from build123d import *

# Parameters (mm, degrees)
SKETCH1_R           = 19.05
BOSS_EXTRUDE1_DEPTH = 5.08
SKETCH3_R           = 7.5
BOSS_EXTRUDE2_DEPTH = 7.62
CUT_EXTRUDE1_DEPTH  = 7.62
SKETCH5_R           = 15.494
CUT_EXTRUDE2_DEPTH  = 3.81


with BuildPart() as part:
    # Sketch1 → Boss-Extrude1 (new body)
    with BuildSketch(Plane(origin=(0, 0, 0), x_dir=(1, 0, 0), z_dir=(0, 1, 0))):
        with Locations(Location((0, 0, 0), (0, 0, 270))):
            Circle(SKETCH1_R)
    extrude(amount=BOSS_EXTRUDE1_DEPTH)

    # Sketch3 → Boss-Extrude2 (add)
    with BuildSketch(Plane(origin=(0, 5.08, 0), x_dir=(1, 0, 0), z_dir=(0, 1, 0))):
        with Locations(Location((0, 0, 0), (0, 0, 90))):
            Circle(SKETCH3_R)
    extrude(amount=BOSS_EXTRUDE2_DEPTH)

    # Sketch4 → Cut-Extrude1 (cut)
    with BuildSketch(Plane(origin=(0, 12.7, 0), x_dir=(1, 0, 0), z_dir=(0, 1, 0))):
        Polygon((4.67653718, 0), (2.33826859, 4.05), (-2.33826859, 4.05), (-4.67653718, 0), (-2.33826859, -4.05), (2.33826859, -4.05), align=None)
    extrude(amount=-CUT_EXTRUDE1_DEPTH, mode=Mode.SUBTRACT)

    # Sketch5 → Cut-Extrude2 (cut)
    with BuildSketch(Plane.XZ):
        with Locations(Location((0, 0, 0), (0, 0, 270))):
            Circle(SKETCH5_R)
    extrude(amount=-CUT_EXTRUDE2_DEPTH, mode=Mode.SUBTRACT)


solid = part.part
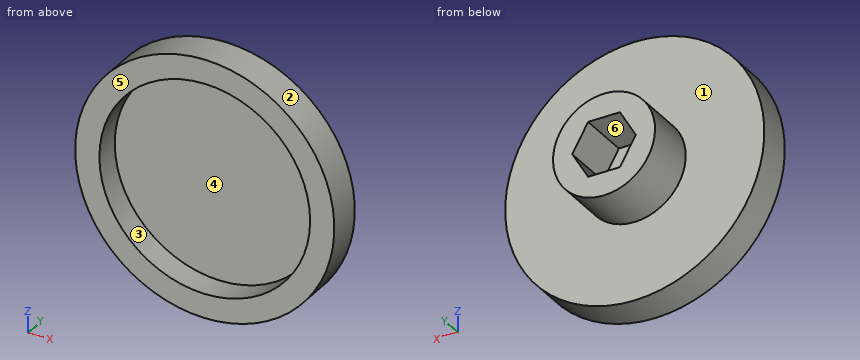
The listing builds one solid part. Answer for the finished solid, in the listing's coordinates (mm). Face numbers are marked on the shaded views. A direction names the side the tool comes from. Coordinates: 2 decimals unless noted, no trailing zeros. Loops run counter-clockwise (first coordinate to the right, second up) from the corner with the lowest first, then second, coordinate; pieces in that order, holes last.
1) Find section A-A on y = 8. Write down the section's boundary in (x, z).
2) Flat-ended cylindrical pins translate along their axes: pin 1 Ø1.5 at (y, z) = (3.5, -0.5) entering from -X; pin 2 Ø1.4 at (x, y) = (-0.5, 7.5) entering from -Z; pin 3 Ø15.5 at (x, z) = (3.5, -6.5) entering from -Y; pin 4 Ø9 at (x, z) = (-2, 1.5) entering from +Y. Find the tip coordinate at first contact, or state that the pin passes through.
3) Find section D-D on x = 11.5. Write down the section's boundary in (y, z), then the cut area to 3 significant figures.
4) Find the intervals of material crossed by L1, parallel to X at y = 2.5, z = 0; L2, parallel to Y at x = -5, z = 9; L3, parallel to Z at x = 14, y = 1.75, in increasing order.
5) Find section B-B on x = 0. Write down the section's boundary in (y, z), then the cut area to 3 significant figures.
6) Determine the mould class of the marked faces 1, 2 and 3 for opening direction Z: pulls with the +Z half, pulls with the -Z half, needs draft (parallel to the pull), parting line crosses it, or undercut.
7) A tool of negligible diameter and unlimited length cuts with its end or side. For the marked faces 4, 5 and 6, from which of +Z, -Z, +X, -X, +Y, -Y can it reach the whole face along a straight path? Write none if from no direction.
8) Find section C-C on z = 14.5. Write down the section's boundary in (x, y).
Values:
1. outline: circle Ø15 at (0, 0); hole (-4.68, 0) - (-2.34, -4.05) - (2.34, -4.05) - (4.68, 0) - (2.34, 4.05) - (-2.34, 4.05) - close
2. pin 1: stops at x = -19.05
2. pin 2: stops at z = -7.5
2. pin 3: stops at y = 3.81
2. pin 4: stops at y = 12.7
3. outline: (0, -15.19) - (5.08, -15.19) - (5.08, 15.19) - (0, 15.19) - (0, 10.38) - (3.81, 10.38) - (3.81, -10.38) - (0, -10.38) - close
3. area: 75.2 mm2
4. L1: x = -19.05 to -15.49, 15.49 to 19.05
4. L2: y = 3.81 to 5.08
4. L3: z = -12.92 to -6.64, 6.64 to 12.92
5. outline: (0, -19.05) - (5.08, -19.05) - (5.08, -7.5) - (12.7, -7.5) - (12.7, -4.05) - (5.08, -4.05) - (5.08, 4.05) - (12.7, 4.05) - (12.7, 7.5) - (5.08, 7.5) - (5.08, 19.05) - (0, 19.05) - (0, 15.49) - (3.81, 15.49) - (3.81, -15.49) - (0, -15.49) - close
5. area: 128 mm2
6. face 1: needs draft
6. face 2: parting line crosses it
6. face 3: undercut
7. face 4: -Y
7. face 5: +Z, -Z, +X, -X, -Y
7. face 6: +Y
8. outline: (-12.36, 0) - (-5.46, 0) - (-5.46, 3.81) - (5.46, 3.81) - (5.46, 0) - (12.36, 0) - (12.36, 5.08) - (-12.36, 5.08) - close
